Check sheet for the modelled part. Datum: model origin and axes. Units: mm. A direction names the side the tool comes from. Coordinates: 2 decimals unless noted, no trailing zeros. Order: outer loops, then holes, each group sorted by start corner. A loop starts at its lowest first (then second) coordinate and runs counter-clockwise, first axis right, second up.
from build123d import *

# Parameters (mm, degrees)
SKETCH1_W             = 75
SKETCH1_H             = 55
BODY_DEPTH            = 10
SHELL1_T              = -2
SKETCH2_R             = 3.25
INSERTS_SUPPORT_DEPTH = 3
SKETCH3_R             = 1.6
INSERTS_HOLES_DEPTH   = 4


with BuildPart() as part:
    # Sketch1 → Body (new body)
    with BuildSketch(Plane(origin=(0, 0, 0), x_dir=(1, 0, 0), z_dir=(0, 1, 0))):
        Rectangle(SKETCH1_W, SKETCH1_H)
    extrude(amount=BODY_DEPTH)

    # Shell1
    shell1_openings = [part.faces().sort_by_distance(p)[0] for p in [
        (0, 10, 0),
    ]]
    offset(amount=SHELL1_T, openings=shell1_openings, kind=Kind.INTERSECTION)

    # Sketch2 → Inserts_Support (add)
    with BuildSketch(Plane(origin=(0, 2, 0), x_dir=(1, 0, 0), z_dir=(0, 1, 0))):
        with Locations(Location((-25, 20, 0), (0, 0, 270))):
            Circle(SKETCH2_R)
        with Locations(Location((25, 20, 0), (0, 0, 270))):
            Circle(SKETCH2_R)
        with Locations(Location((25, -20, 0), (0, 0, 270))):
            Circle(SKETCH2_R)
        with Locations(Location((-25, -20, 0), (0, 0, 270))):
            Circle(SKETCH2_R)
    extrude(amount=INSERTS_SUPPORT_DEPTH)

    # Sketch3 → Inserts_Holes (cut)
    with BuildSketch(Plane(origin=(0, 5, 0), x_dir=(1, 0, 0), z_dir=(0, 1, 0))):
        with Locations(Location((-25, 20, 0), (0, 0, 270))):
            Circle(SKETCH3_R)
        with Locations(Location((25, 20, 0), (0, 0, 270))):
            Circle(SKETCH3_R)
        with Locations(Location((25, -20, 0), (0, 0, 270))):
            Circle(SKETCH3_R)
        with Locations(Location((-25, -20, 0), (0, 0, 270))):
            Circle(SKETCH3_R)
    extrude(amount=-INSERTS_HOLES_DEPTH, mode=Mode.SUBTRACT)


solid = part.part
(1) Cross-section at B-B (z = 20). Enter the section's corners in (x, y), and give its area (3 significant figures).
Filled in:
outline: (-37.5, 0) - (37.5, 0) - (37.5, 10) - (35.5, 10) - (35.5, 2) - (28.25, 2) - (28.25, 5) - (26.6, 5) - (26.6, 1) - (23.4, 1) - (23.4, 5) - (21.75, 5) - (21.75, 2) - (-21.75, 2) - (-21.75, 5) - (-23.4, 5) - (-23.4, 1) - (-26.6, 1) - (-26.6, 5) - (-28.25, 5) - (-28.25, 2) - (-35.5, 2) - (-35.5, 10) - (-37.5, 10) - close
area: 195 mm2
(2) Cross-section at D-D (y = 7.75). Enter the section's corners in (x, z).
Filled in:
outline: (-37.5, -27.5) - (37.5, -27.5) - (37.5, 27.5) - (-37.5, 27.5) - close; hole (-35.5, -25.5) - (35.5, -25.5) - (35.5, 25.5) - (-35.5, 25.5) - close
(3) Release check for a two-part mould opening along Z. For faces 3 (the flat face through (-3, 10, 26)), 4 (the flat face through (-1, 5, -27.5)), 5 (the cylindrical face through (-26.978, 3.479, -22.579)), 6 (the flat face through (-26.4, 5, 21.4)) record: +Z half, -Z half, draft (parallel to the pull), parting line (faces both ways), or undercut.
Filled in:
face 3: draft
face 4: -Z half
face 5: undercut
face 6: undercut
(4) Tool access check on faces 1 (the flat face through (-37.5, 5, 0)), 2 (the cylindrical face through (-23.92, 3.03, 18.82)). Record the directions out of +Z, -Z, +X, -X, +Y, -Y that give a thin tool (end or side, any length) a straight path to the whole face; none if there is none.
Filled in:
face 1: +Z, -Z, -X, +Y, -Y
face 2: +Y
(5) Go/stop test with flat-tipped pins: P1, Ø2.5, axis at x = -26, z = -19.5, coming from the +Y side; P2, Ø12, axis at x = 6.5, z = 17, coming from the +Y side. Record where each tip stops, or that it passes through.
Filled in:
P1: stops at y = 5
P2: stops at y = 2
(6) Cross-section at A-A (y = 3.25). Count the separate pieces of the cut face and the enclosed holes in it, and give its area (3 significant figures).
Filled in:
separate pieces: 5
enclosed holes: 5
area: 605 mm2
(7) Thickness scan on probe 1 along X at (y, z) = (3.15, -20); probe 2 along Z at (x, y) = (-32, 7.75); probe 3 along X at (y, z) = (8.5, 4.5). Record the ranges inside material, lowest first.
Filled in:
probe 1: x = -37.5 to -35.5, -28.25 to -26.6, -23.4 to -21.75, 21.75 to 23.4, 26.6 to 28.25, 35.5 to 37.5
probe 2: z = -27.5 to -25.5, 25.5 to 27.5
probe 3: x = -37.5 to -35.5, 35.5 to 37.5
(8) Cross-section at C-C (x = -21). Enter the section's corners in (y, z).
Filled in:
outline: (0, -27.5) - (10, -27.5) - (10, -25.5) - (2, -25.5) - (2, 25.5) - (10, 25.5) - (10, 27.5) - (0, 27.5) - close
